from build123d import *

# Parameters (mm, degrees)
SKETCH1_R           = 2.05
BOSS_EXTRUDE1_DEPTH = 3.5
FILLET1_R           = 5
SKETCH2_R           = 4.55
BOSS_EXTRUDE2_DEPTH = 1
SKETCH3_R           = 4.55
SKETCH3_R_2         = 2.05
BOSS_EXTRUDE3_DEPTH = 2.5
FILLET2_R           = 1


with BuildPart() as part:
    # Sketch1 → Boss-Extrude1 (new body)
    with BuildSketch(Plane.XY):
        with BuildLine():
            ThreePointArc((82.7, -2.05), (85.917335854, 5.717335854), (78.15, 2.5))
            Line((78.15, 2.5), (2.05, 2.5))
            ThreePointArc((2.05, 2.5), (-5.717335854, 5.717335854), (-2.5, -2.05))
            Line((-2.5, -2.05), (-2.5, -78.15))
            ThreePointArc((-2.5, -78.15), (-5.717335854, -85.917335854), (2.05, -82.7))
            Line((2.05, -82.7), (78.15, -82.7))
            ThreePointArc((78.15, -82.7), (85.917335854, -85.917335854), (82.7, -78.15))
            Line((82.7, -78.15), (82.7, -2.05))
        make_face()
        with Locations((82.7, -82.7)):
            Circle(SKETCH1_R, mode=Mode.SUBTRACT)
        with Locations((-2.5, -82.7)):
            Circle(SKETCH1_R, mode=Mode.SUBTRACT)
        with Locations((82.7, 2.5)):
            Circle(SKETCH1_R, mode=Mode.SUBTRACT)
        with Locations((-2.5, 2.5)):
            Circle(SKETCH1_R, mode=Mode.SUBTRACT)
    extrude(amount=BOSS_EXTRUDE1_DEPTH)

    # Fillet1
    fillet1_edges = [part.edges().sort_by_distance(p)[0] for p in [
        (2.05, 2.5, 1.75),
        (78.15, 2.5, 1.75),
        (82.7, -2.05, 1.75),
        (82.7, -78.15, 1.75),
        (78.15, -82.7, 1.75),
        (2.05, -82.7, 1.75),
        (-2.5, -78.15, 1.75),
        (-2.5, -2.05, 1.75),
    ]]
    fillet(fillet1_edges, radius=FILLET1_R)

    # Sketch2 → Boss-Extrude2 (add)
    with BuildSketch(Plane(origin=(0, 0, 0), x_dir=(-1, 0, 0), z_dir=(0, 0, -1))):
        with Locations((-82.7, 2.5)):
            Circle(SKETCH2_R)
        with Locations((2.5, 2.5)):
            Circle(SKETCH2_R)
        with Locations((2.5, -82.7)):
            Circle(SKETCH2_R)
        with Locations((-82.7, -82.7)):
            Circle(SKETCH2_R)
    extrude(amount=-BOSS_EXTRUDE2_DEPTH)

    # Sketch3 → Boss-Extrude3 (add)
    with BuildSketch(Plane.XY.offset(3.5)):
        with Locations((-2.5, 2.5)):
            Circle(SKETCH3_R)
        with Locations((-2.5, 2.5)):
            Circle(SKETCH3_R_2, mode=Mode.SUBTRACT)
        with Locations((82.7, 2.5)):
            Circle(SKETCH3_R)
        with Locations((82.7, 2.5)):
            Circle(SKETCH3_R_2, mode=Mode.SUBTRACT)
        with Locations((82.7, -82.7)):
            Circle(SKETCH3_R)
        with Locations((82.7, -82.7)):
            Circle(SKETCH3_R_2, mode=Mode.SUBTRACT)
        with Locations((-2.5, -82.7)):
            Circle(SKETCH3_R)
        with Locations((-2.5, -82.7)):
            Circle(SKETCH3_R_2, mode=Mode.SUBTRACT)
    extrude(amount=BOSS_EXTRUDE3_DEPTH)

    # Fillet2
    fillet2_edges = [part.edges().sort_by_distance(p)[0] for p in [
        (-4.55, 2.5, 6),
        (80.65, 2.5, 6),
        (80.65, -82.7, 6),
        (-4.55, -82.7, 6),
    ]]
    fillet(fillet2_edges, radius=FILLET2_R)


solid = part.part
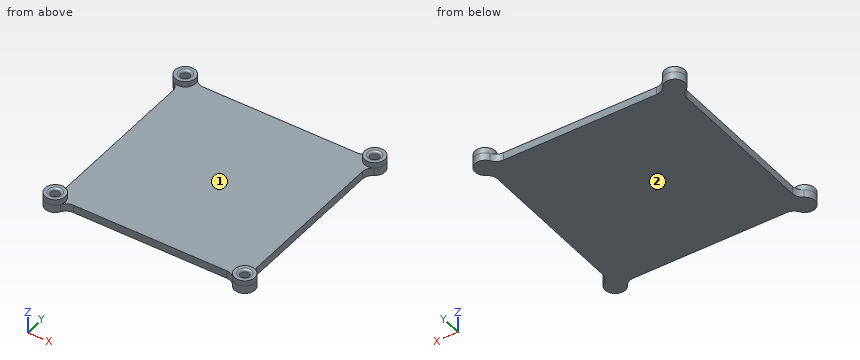
Verification items for the finished model (mm, model axes). Face numbers are marked on the shaded views. A direction names the side the tool comes from. Coordinates: 2 decimals unless noted, no trailing zeros. Order: outer loops, then holes, each group sorted by start corner. A loop starts at its lowest first (then second) coordinate and runs counter-clockwise, first axis right, second up. Notation, with made-up numbers: M 60,53.5 L 80,53.5 A22 cw 80,87.5 Z; hole C -25.5,-39.5 d10. An arc over 180 degrees is marked long. One line per item, written item: value. Start each with the question number.
Item 1: Depth check by flat-ended pin: P1, Ø3, axis at y = -23.5, z = 1.5, coming from the -X side; P2, Ø2, axis at x = -3, y = 3, coming from the +Z side; P3, Ø12, axis at x = 57.5, y = -46.5, coming from the +Z side. Enter the tip coordinate at first touch or a pass-through.
Item 2: Sectioned sample at B-B on y = -62.5. Record the cut outline in (x, z).
Item 3: Sectioned sample at C-C on x = 49. Record the cut outline in (y, z).
Item 4: Sectioned sample at A-A on z = 2.45. Record the cut outline in (x, y), then the cut area to 3 significant figures.
Item 5: Access from +Z, -Z, +X, -X, +Y, -Y to the whole of each face (thin tool, end or side, straight path). Record for the marked faces 1 and 2.
Item 6: Thickness scan on probe 1 along X at (y, z) = (-82.7, 4.2); probe 2 along Y at (x, z) = (28.5, 2); probe 3 along X at (y, z) = (-33, 1). Record the ranges inside material, lowest first.
Calculated:
1. P1: x = -2.5
1. P2: z = 1
1. P3: z = 3.5
2. outline: M -2.5,0 L 82.7,0 L 82.7,3.5 L -2.5,3.5 Z
3. outline: M -82.7,0 L 2.5,0 L 2.5,3.5 L -82.7,3.5 Z
4. outline: M -4.88,-78.82 A4.55 ccw long 1.38,-85.08 A5 cw 5.64,-82.7 L 74.56,-82.7 A5 cw 78.82,-85.08 A4.55 ccw long 85.08,-78.82 A5 cw 82.7,-74.56 L 82.7,-5.64 A5 cw 85.08,-1.38 A4.55 ccw long 78.82,4.88 A5 cw 74.56,2.5 L 5.64,2.5 A5 cw 1.38,4.88 A4.55 ccw long -4.88,-1.38 A5 cw -2.5,-5.64 L -2.5,-74.56 A5 cw Z; hole C -2.5,-82.7 d4.1; hole C -2.5,2.5 d4.1; hole C 82.7,-82.7 d4.1; hole C 82.7,2.5 d4.1
4. area: 7,420 mm^2
5. face 1: +Z
5. face 2: -Z, +X, -X, +Y, -Y
6. probe 1: -7.05 to -4.55, -0.45 to 2.05, 78.15 to 80.65, 84.75 to 87.25
6. probe 2: -82.7 to 2.5
6. probe 3: -2.5 to 82.7
